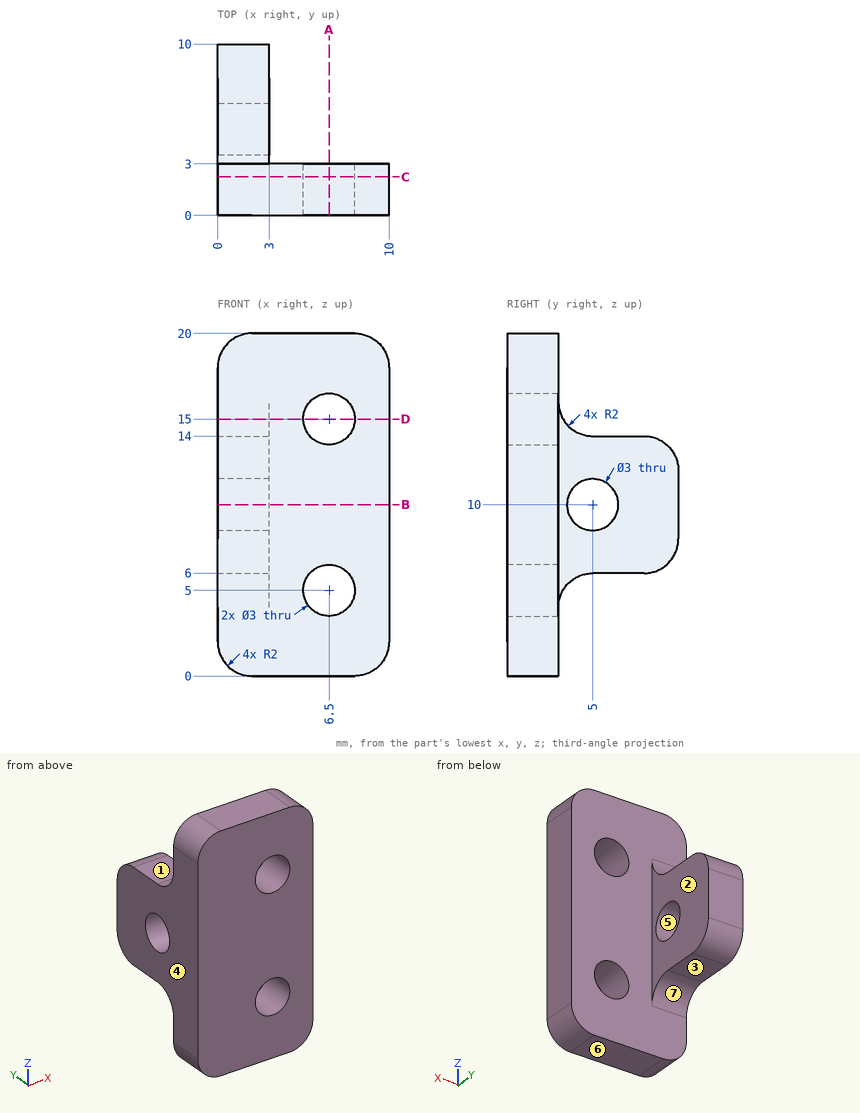
Geometry check sheet. Reference: drawing and pictorial views, mm from the part's lowest x, y, z. A direction names the side the tool comes from. Coordinates: 2 decimals unless noted, no trailing zeros. Order: outer loops, then holes, each group sorted by start corner. A loop starts at its lowest first (then second) coordinate and runs counter-clockwise, first axis right, second up. Notation, with made-up numbers: M 48,25 L 100,25 A17 ccw 100,34 Z; hole C 32.25,64 d1. An arc over 180 degrees is marked long. Return JSON: item names as keys, results as strings.
1) Gauge pin test, flat ends, axial feed: pin 1 (2.5 mm diameter, centred on y = 5, z = 10, fed in from +X); pin 2 (1.5 mm diameter, centred on x = 2, y = 6.5, fed in from -Z); pin 3 (5.5 mm diameter, centred on y = 6, z = 7.5, fed in from +X); pin 4 (3.5 mm diameter, centred on x = 2, y = 7, fed in from +Z). Record the tip position at first contact, or that the pin passes through.
Answer list:
{"pin 1": "through", "pin 2": "z = 6", "pin 3": "x = 3", "pin 4": "z = 14"}
2) Cross-section at B-B, the plane z = 10. Record the boundary of the cut face in (x, y), and give its area (3 significant figures).
Answer list:
{"outline": "M 0,0 L 10,0 L 10,3 L 3,3 L 3,3.5 L 0,3.5 Z; M 0,6.5 L 3,6.5 L 3,10 L 0,10 Z", "area": "42.0 mm2"}
3) Access from +Z, -Z, +X, -X, +Y, -Y to the whole of each face (thin tool, end or side, straight path). Record for the marked faces 1, 2, 3 and 4.
Answer list:
{"face 1": "+Z, +X, -X, +Y", "face 2": "+Z, -Z, +X, +Y", "face 3": "-Z, +X, -X, +Y", "face 4": "+Z, -Z, -X, +Y, -Y"}
4) Cross-section at C-C, the plane y = 2.25. Record the boundary of the cut face in (x, z), and give its area (3 significant figures).
Answer list:
{"outline": "M 0,2 A2 ccw 2,0 L 8,0 A2 ccw 10,2 L 10,18 A2 ccw 8,20 L 2,20 A2 ccw 0,18 Z; hole C 6.5,5 d3; hole C 6.5,15 d3", "area": "182 mm2"}
5) Release check for a two-part mould opening along Y. For the marked faces 5, 6 and 7 record: +Y half, -Y half, draft (parallel to the pull), parting line (faces both ways), or undercut.
Answer list:
{"face 5": "undercut", "face 6": "draft", "face 7": "+Y half"}
6) Thickness scan on L1, parallel to X at y = 1.85, z = 5; L2, parallel to Z at x = 7.5, y = 2.5; L3, parallel to Y at x = 1.1, z = 10. Record the ranges inside material, lowest first. Write a range as [from, to].
Answer list:
{"L1": "[0, 5], [8, 10]", "L2": "[0, 3.88], [6.12, 13.88], [16.12, 20]", "L3": "[0, 3.5], [6.5, 10]"}
7) Cross-section at D-D, the plane z = 15. Record the boundary of the cut face in (x, y).
Answer list:
{"outline": "M 0,0 L 5,0 L 5,3 L 3,3 L 3,3.27 L 0,3.27 Z; M 8,0 L 10,0 L 10,3 L 8,3 Z"}
8) Cross-section at A-A, the plane x = 6.5. Record the boundary of the cut face in (y, z).
Answer list:
{"outline": "M 0,0 L 3,0 L 3,3.5 L 0,3.5 Z; M 0,6.5 L 3,6.5 L 3,13.5 L 0,13.5 Z; M 0,16.5 L 3,16.5 L 3,20 L 0,20 Z"}
